Geometry: final body of the model. Coordinates: model frame, mm. A direction names the side the tool comes from. Round coordinates to 2 decimals unless told otherwise and drop trailing zeros. Write each loop counter-clockwise with the first axis right and the second up, starting at its lowest first coordinate (ties: lowest second). Pieces come first, ordered by that corner, then holes. Notation, with made-up numbers: (19, -16.5) - (71, -16.5) arc R27 ccw to (71, 2.5) - close; hole circle Ø3 at (-20.75, 42). An arc over 180 degrees is marked (long way). Write each question's results on one line, items separated by ' | '.
from build123d import *

# Parameters (mm, degrees)
SKETCH1_W           = 33.8328
SKETCH1_H           = 25.4
BOSS_EXTRUDE1_DEPTH = 1.524
FILLET1_R           = 1.8542
SKETCH2_R           = 1.1938
SKETCH2_R_2         = 0.8001
CUT_EXTRUDE1_DEPTH  = 1.524
SKETCH3_W           = 25.4
SKETCH3_H           = 25.4
BOSS_EXTRUDE2_DEPTH = 23.876
FILLET2_R           = 0.762
BOSS_EXTRUDE3_DEPTH = 2.032
SKETCH5_W           = 13.97
SKETCH5_H           = 6.858
BOSS_EXTRUDE4_DEPTH = 1.9304
FILLET3_R           = 1.524
SKETCH6_R           = 0.635
BOSS_EXTRUDE5_DEPTH = 4.064
SKETCH7_R           = 1.576094172
BOSS_EXTRUDE6_DEPTH = 0.762
FILLET4_R           = 0.5588
CUT_EXTRUDE2_DEPTH  = 0.762


with BuildPart() as part:
    # Sketch1 → Boss-Extrude1 (new body)
    with BuildSketch(Plane(origin=(0, 0, 0), x_dir=(1, 0, 0), z_dir=(0, 1, 0))):
        Rectangle(SKETCH1_W, SKETCH1_H)
    extrude(amount=BOSS_EXTRUDE1_DEPTH)

    # Fillet1
    fillet1_edges = [part.edges().sort_by_distance(p)[0] for p in [
        (16.9164, 0.762, 12.7),
        (-16.9164, 0.762, 12.7),
        (-16.9164, 0.762, -12.7),
        (16.9164, 0.762, -12.7),
    ]]
    fillet(fillet1_edges, radius=FILLET1_R)

    # Sketch2 → Cut-Extrude1 (cut)
    with BuildSketch(Plane(origin=(0, 1.524, 0), x_dir=(1, 0, 0), z_dir=(0, 1, 0))):
        with Locations(Location((15.0622, -10.8458, 0), (0, 0, 270))):
            Circle(SKETCH2_R)
        with Locations(Location((15.0622, 10.8458, 0), (0, 0, 270))):
            Circle(SKETCH2_R)
        with Locations(Location((-15.0368, 10.8458, 0), (0, 0, 270))):
            Circle(SKETCH2_R)
        with Locations(Location((-15.0368, -10.8458, 0), (0, 0, 270))):
            Circle(SKETCH2_R)
        with Locations(Location((-15.0368, 0, 0), (0, 0, 270))):
            Circle(SKETCH2_R_2)
        with BuildLine():
            Line((15.4559, -0.8001), (14.6685, -0.8001))
            ThreePointArc((14.6685, -0.8001), (13.8684, 0), (14.6685, 0.8001))
            Line((14.6685, 0.8001), (15.4559, 0.8001))
            ThreePointArc((15.4559, 0.8001), (16.256, 0), (15.4559, -0.8001))
        make_face()
    extrude(amount=-CUT_EXTRUDE1_DEPTH, mode=Mode.SUBTRACT)

    # Sketch3 → Boss-Extrude2 (add)
    with BuildSketch(Plane(origin=(0, 1.524, 0), x_dir=(1, 0, 0), z_dir=(0, 1, 0))):
        Rectangle(SKETCH3_W, SKETCH3_H)
    extrude(amount=BOSS_EXTRUDE2_DEPTH)

    # Fillet2
    fillet2_edges = [part.edges().sort_by_distance(p)[0] for p in [
        (12.7, 13.462, 12.7),
        (-12.7, 13.462, 12.7),
        (-12.7, 13.462, -12.7),
        (12.7, 13.462, -12.7),
    ]]
    fillet(fillet2_edges, radius=FILLET2_R)

    # Sketch4 → Boss-Extrude3 (add)
    with BuildSketch(Plane(origin=(0, 25.4, 0), x_dir=(1, 0, 0), z_dir=(0, 1, 0))):
        Polygon((0, -0.4826), (0, -3.9878), (6.985, -3.9878), (10.414, -3.9878), (10.414, -0.4826), align=None)
        Polygon((-6.985, -3.9878), (0, -3.9878), (0, -0.4826), (-10.414, -0.4826), (-10.414, -3.9878), align=None)
    extrude(amount=BOSS_EXTRUDE3_DEPTH)

    # Sketch5 → Boss-Extrude4 (add)
    with BuildSketch(Plane(origin=(0, 25.4, 0), x_dir=(1, 0, 0), z_dir=(0, 1, 0))):
        with Locations((0, -7.4168)):
            Rectangle(SKETCH5_W, SKETCH5_H)
    extrude(amount=BOSS_EXTRUDE4_DEPTH)

    # Fillet3
    fillet3_edges = [part.edges().sort_by_distance(p)[0] for p in [
        (6.985, 26.3652, 10.8458),
        (-6.985, 26.3652, 10.8458),
    ]]
    fillet(fillet3_edges, radius=FILLET3_R)

    # Sketch6 → Boss-Extrude5 (add)
    with BuildSketch(Plane(origin=(0, 0, 0.4826), x_dir=(-1, 0, 0), z_dir=(0, 0, -1))):
        with Locations(Location((-4.8895, 26.555352192, 0), (0, 0, 180))):
            Circle(SKETCH6_R)
        with Locations(Location((3.4925, 26.555352192, 0), (0, 0, 180))):
            Circle(SKETCH6_R)
        with Locations(Location((4.8895, 26.555352192, 0), (0, 0, 180))):
            Circle(SKETCH6_R)
        with Locations(Location((2.0955, 26.555352192, 0), (0, 0, 180))):
            Circle(SKETCH6_R)
        with Locations(Location((-2.0955, 26.555352192, 0), (0, 0, 180))):
            Circle(SKETCH6_R)
        with Locations(Location((0.6985, 26.555352192, 0), (0, 0, 180))):
            Circle(SKETCH6_R)
        with Locations(Location((-3.4925, 26.555352192, 0), (0, 0, 180))):
            Circle(SKETCH6_R)
        with Locations(Location((-0.6985, 26.555352192, 0), (0, 0, 180))):
            Circle(SKETCH6_R)
        with Locations(Location((-6.2865, 26.555352192, 0), (0, 0, 180))):
            Circle(SKETCH6_R)
        with Locations(Location((6.2865, 26.555352192, 0), (0, 0, 180))):
            Circle(SKETCH6_R)
    extrude(amount=BOSS_EXTRUDE5_DEPTH)

    # Sketch7 → Boss-Extrude6 (add)
    with BuildSketch(Plane(origin=(0, 27.432, 0), x_dir=(1, 0, 0), z_dir=(0, 1, 0))):
        with Locations(Location((7.385275371, -2.2352, 0), (0, 0, 90))):
            Circle(SKETCH7_R)
        with Locations(Location((-7.385275371, -2.2352, 0), (0, 0, 90))):
            Circle(SKETCH7_R)
    extrude(amount=BOSS_EXTRUDE6_DEPTH)

    # Fillet4
    fillet4_edges = [part.edges().sort_by_distance(p)[0] for p in [
        (7.385275371, 28.194, 3.811294172),
        (-7.385275371, 28.194, 3.811294172),
    ]]
    fillet(fillet4_edges, radius=FILLET4_R)

    # Sketch8 → Cut-Extrude2 (cut)
    with BuildSketch(Plane(origin=(0, 28.194, 0), x_dir=(1, 0, 0), z_dir=(0, 1, 0))):
        Polygon((7.537675371, -1.4732), (7.537675371, -2.0828), (8.147275371, -2.0828), (8.147275371, -2.3876), (7.537675371, -2.3876), (7.537675371, -2.9972), (7.232875371, -2.9972), (7.232875371, -2.3876), (6.623275371, -2.3876), (6.623275371, -2.0828), (7.232875371, -2.0828), (7.232875371, -1.4732), align=None)
        Polygon((-7.232875371, -2.3876), (-6.623275371, -2.3876), (-6.623275371, -2.0828), (-7.232875371, -2.0828), (-7.232875371, -1.4732), (-7.537675371, -1.4732), (-7.537675371, -2.0828), (-8.147275371, -2.0828), (-8.147275371, -2.3876), (-7.537675371, -2.3876), (-7.537675371, -2.9972), (-7.232875371, -2.9972), align=None)
    extrude(amount=-CUT_EXTRUDE2_DEPTH, mode=Mode.SUBTRACT)


solid = part.part
Q1. Section query B-B, the plane y = 17.75. Return loops of the section in (x, z), plus the area to 3 significant figures.
Answer block:
outline: (-12.7, -11.94) arc R0.76 ccw to (-11.94, -12.7) - (11.94, -12.7) arc R0.76 ccw to (12.7, -11.94) - (12.7, 11.94) arc R0.76 ccw to (11.94, 12.7) - (-11.94, 12.7) arc R0.76 ccw to (-12.7, 11.94) - close | area: 645 mm2
Q2. Ray query, line 1 along X through (y, z) = (1.05, 0); line 2 along Y through (x, z) = (2, -3.25); line 3 along Y through (x, z) = (0, -7). Return the intervals inside material, ascending.
Answer block:
line 1: -16.92 to -15.84, -14.24 to 13.87, 16.26 to 16.92 | line 2: 0 to 25.4, 25.93 to 27.18 | line 3: 0 to 25.4
Q3. Pin query (flat end, axial travel): pin 1 (1.5 mm diameter, centred on y = 7.5, z = -4, fed in from -X); pin 2 (0.5 mm diameter, centred on y = 27.5, z = 1.5, fed in from -X); pin 3 (0.7 mm diameter, centred on x = -8, y = 28, fed in from -Z). Return the tip coordinate at first contact, or that it passes through.
Answer block:
pin 1: x = -12.7 | pin 2: x = -10.41 | pin 3: z = 0.72
Q4. Section query C-C, the plane z = -10.25. Return loops of the section in (x, y), plus the area to 3 significant figures.
Answer block:
outline: (-16.92, 0) - (-16.07, 0) - (-16.07, 1.52) - (-16.92, 1.52) - close; (-14, 0) - (14.03, 0) - (14.03, 1.52) - (12.7, 1.52) - (12.7, 25.4) - (-12.7, 25.4) - (-12.7, 1.52) - (-14, 1.52) - close; (16.1, 0) - (16.92, 0) - (16.92, 1.52) - (16.1, 1.52) - close | area: 652 mm2
Q5. Access query for faces 1 (the cylindrical face through (16.256, 0.773, -0.018)), 2 (the flat face through (6.985, 26, 7)), 3 (the flat face through (-3.5, 26.5, -3.581)), 4 (the flat face through (10.414, 26, 2)). Directions: +Z, -Z, +X, -X, +Y, -Y. A direction counts if a zero-diameter tool reaches every point of the face in a straight line with its end or side. Return the directions, or none.
Answer block:
face 1: +Y, -Y | face 2: +Z, +X, +Y | face 3: -Z, +X, -X, +Y | face 4: +Z, -Z, +X, +Y
Q6. Section query D-D, the plane z = -3. Give the number of separate pieces and of enclosed holes in the cut face, plus the area to 3 significant figures.
Answer block:
separate pieces: 11 | enclosed holes: 0 | area: 671 mm2
Q7. Section query A-A, the plane z = -7. Return loops of the section in (x, y), plus the area to 3 significant figures.
Answer block:
outline: (-16.92, 0) - (16.92, 0) - (16.92, 1.52) - (12.7, 1.52) - (12.7, 25.4) - (-12.7, 25.4) - (-12.7, 1.52) - (-16.92, 1.52) - close | area: 658 mm2
Q8. Mould query, pull axis Z, two halves, no side actions, for faces 5 (the flat face through (-2, 27, -3.581)), 6 (the flat face through (-16.916, 1, 0)), 7 (the cylindrical face through (-14.244, 0.773, -0.104)). Classes: pulls with the +Z half, pulls with the -Z half, needs draft (parallel to the pull), parting line crosses it, or undercut.
Answer block:
face 5: pulls with the -Z half | face 6: needs draft | face 7: undercut
